from build123d import *

# Parameters (mm, degrees)
EXTRUDE_1_DEPTH          = 25
CUT_EXTRUDE_2_DEPTH      = 52.23475383
CUT_EXTRUDE_2_DEPTH_BACK = 52.23475383
SKETCH_2_R               = 5
CUT_EXTRUDE_3_DEPTH      = 52.23475383
CUT_EXTRUDE_3_DEPTH_BACK = 52.23475383
SKETCH_3_R               = 5
CHAMFER_1_SIZE           = 5


with BuildPart() as part:
    # 草圖1 → 填料-伸長1 (new body)
    with BuildSketch(Plane(origin=(0, 0, 0), x_dir=(1, 0, 0), z_dir=(0, 1, 0))):
        Polygon((0, 0), (20, 20), (40, 0), (20, -20), align=None)
    extrude(amount=EXTRUDE_1_DEPTH)

    # 草圖2 → 除料-伸長2 (cut, two sides: drawn at the far end of the back side and taken through both)
    with BuildSketch(Plane(origin=(0, 0, 0), x_dir=(0, 0, -1), z_dir=(1, 0, 0)).offset(-CUT_EXTRUDE_2_DEPTH_BACK)):
        with Locations(Location((0, 6.25, 0), (0, 0, 270.000068755))):
            Circle(SKETCH_2_R)
    extrude(amount=CUT_EXTRUDE_2_DEPTH + CUT_EXTRUDE_2_DEPTH_BACK, mode=Mode.SUBTRACT)

    # 草圖3 → 除料-伸長3 (cut, two sides: drawn at the far end of the back side and taken through both)
    with BuildSketch(Plane.XY.offset(-CUT_EXTRUDE_3_DEPTH_BACK)):
        with Locations(Location((20, 18.75, 0), (0, 0, 90))):
            Circle(SKETCH_3_R)
    extrude(amount=CUT_EXTRUDE_3_DEPTH + CUT_EXTRUDE_3_DEPTH_BACK, mode=Mode.SUBTRACT)

    # 導角1
    # the kernel refuses this chamfer: 5 mm, written as the material it takes off along each edge
    with BuildSketch(Plane(origin=(49.092272399, 0, -9.092272399), x_dir=(0.01944252080601414, 0.9996219169112968, 0.01944252080601414), z_dir=(-0.7071067811865476, 0, 0.7071067811865476)), Plane(origin=(10.907727601, 0, -29.092272399), x_dir=(0.019442520806014316, 0.9996219169112968, -0.01944252080601431), z_dir=(0.7071067811865475, 0, 0.7071067811865476)), Plane(origin=(-9.092272399, 0, 9.092272399), x_dir=(-0.01944252080601397, 0.9996219169112968, -0.019442520806013965), z_dir=(0.7071067811865475, 0, -0.7071067811865476)), Plane(origin=(29.092272399, 0, 29.092272399), x_dir=(-0.019442520806014486, 0.9996219169112968, 0.019442520806014486), z_dir=(-0.7071067811865476, 0, -0.7071067811865476)), Plane(origin=(10.907727601, 25, -29.092272399), x_dir=(-0.7068394360706736, 0.027495876610586313, 0.7068394360706735), z_dir=(0.7071067811865475, 0, 0.7071067811865476))) as chamfer_1_piece_1:
        Polygon((CHAMFER_1_SIZE * 0.999621916911, CHAMFER_1_SIZE * 0.0274958766106), (-CHAMFER_1_SIZE * 0.0274958766106, CHAMFER_1_SIZE * 0.999621916911), (0, 0), align=None)
    extrude(amount=54.001101127, mode=Mode.SUBTRACT)
    with BuildSketch(Plane(origin=(29.092272399, 25, 29.092272399), x_dir=(-0.019442520806014486, -0.9996219169112968, 0.019442520806014486), z_dir=(-0.7071067811865476, 0, -0.7071067811865476)), Plane(origin=(-9.092272399, 25, 9.092272399), x_dir=(-0.01944252080601397, -0.9996219169112968, -0.019442520806013965), z_dir=(0.7071067811865475, 0, -0.7071067811865476)), Plane(origin=(49.092272399, 25, -9.092272399), x_dir=(0.01944252080601414, -0.9996219169112968, 0.01944252080601414), z_dir=(-0.7071067811865476, 0, 0.7071067811865476))) as chamfer_1_piece_2:
        Polygon((CHAMFER_1_SIZE * 0.999621916911, -CHAMFER_1_SIZE * 0.0274958766106), (-CHAMFER_1_SIZE * 0.0274958766106, -CHAMFER_1_SIZE * 0.999621916911), (0, 0), align=None)
    extrude(amount=54.001101127, mode=Mode.SUBTRACT)


solid = part.part
Can you work these out from the model? Positions are in its coordinate system, mm. Round coordinates to 2 decimals unless told otherwise and drop trailing zeros. Order: outer loops, then holes, each group sorted by start corner. A loop starts at its lowest first (then second) coordinate and runs counter-clockwise, first axis right, second up. Notation, with made-up numbers: M -5,88.25 L 25,88.25 A17 ccw 25,111.25 Z; hole C 59.5,9.25 d4. An arc over 180 degrees is marked long. Use a Markdown table: item, result.
1) Imagine slicing it at D-D (x = 32). List the corners of the cut face in (y, z) for me.
Geometry says:
| item | result |
|---|---|
| outline | M 0,-0.93 L 5,-8 L 20,-8 L 25,-0.93 L 25,0.93 L 20,8 L 5,8 L 0,0.93 Z; hole C 6.25,0 d10 |
2) Imagine slicing it at B-B (x = 17). List the corners of the cut face in (y, z) for me.
Geometry says:
| item | result |
|---|---|
| outline | M 0,-9.93 L 5,-17 L 14.75,-17 L 14.75,17 L 5,17 L 0,9.93 Z; M 22.75,-13.11 L 25,-9.93 L 25,9.93 L 22.75,13.11 Z; hole C 6.25,0 d10 |
3) Imagine slicing it at C-C (y = 10.25). List the corners of the cut face in (x, z) for me.
Geometry says:
| item | result |
|---|---|
| outline | M 3,-3 L 20,-20 L 37,-3 Z; M 3,3 L 37,3 L 20,20 Z |
4) If I drill on line 1 along Y through (x, z) = (20, 12); line 2 along Z through (x, y) = (14.5, 6.25); line 3 along Y through (x, z) = (17, -8), over which ranges is the centre line in solid material (lowest first)?
Geometry says:
| item | result |
|---|---|
| line 1 | y = 0 to 13.75, 23.75 to 25 |
| line 2 | z = -14.5 to -5, 5 to 14.5 |
| line 3 | y = 0 to 14.75, 22.75 to 25 |
5) I'm going to push flat-ended pins straight in: P1, Ø3, axis at x = 17.5, y = 5, coming from the +Z side; P2, Ø2, axis at x = 6, y = 9.5, coming from the +Z side; P3, Ø1, axis at x = 26.5, y = 19, coming from the -Z side. Where does each tip first touch, or does it pass through?
Geometry says:
| item | result |
|---|---|
| P1 | stops at z = 19 |
| P2 | stops at z = 7 |
| P3 | stops at z = -14 |
6) Imagine slicing it at A-A (z = 0.5). List the corners of the cut face in (x, y) for me.
Geometry says:
| item | result |
|---|---|
| outline | M 0.5,11.22 L 39.5,11.22 L 39.5,20 L 32.43,25 L 7.57,25 L 0.5,20 Z; M 5.77,1.28 L 7.57,0 L 32.43,0 L 34.23,1.28 Z; hole C 20,18.75 d10 |
7) If we mould it in two halves opening along X, with no side actions, what happens to faces 1 (the face through (19.78, 13.755, -0.28)), 2 (the face through (27.05, 2.53, 9.46)), 3 (the face through (20, 0, 0))? For each: +X half, -X half, draft (parallel to the pull), parting line (faces both ways), or undercut.
Geometry says:
| item | result |
|---|---|
| face 1 | undercut |
| face 2 | +X half |
| face 3 | draft |
